```python
from build123d import *

# Parameters (mm, degrees)
SKETCH_W      = 300
SKETCH_H      = 300
PAD_DEPTH     = 30
SKETCH001_W   = 300
SKETCH001_H   = 300
SKETCH001_W_2 = 240
SKETCH001_H_2 = 240
PAD001_DEPTH  = 100


with BuildPart() as body:
    # Sketch → Pad (new body)
    with BuildSketch(Plane.XY):
        with Locations((150, 150)):
            Rectangle(SKETCH_W, SKETCH_H)
    extrude(amount=PAD_DEPTH)


with BuildPart() as body001:
    # Sketch001 (on Face6 of Pad) → Pad001 (new body)
    with BuildSketch(Plane.XY.offset(30)):
        with Locations((150, 150)):
            Rectangle(SKETCH001_W, SKETCH001_H)
        with Locations((150, 150)):
            Rectangle(SKETCH001_W_2, SKETCH001_H_2, mode=Mode.SUBTRACT)
    extrude(amount=PAD001_DEPTH)

    # Boolean: union Body
    add(body.part)


solid = body001.part
```
Input: part model. Units: mm. Frame: model coordinates. A direction names the side the tool comes from. Round coordinates to 2 decimals unless told otherwise and drop trailing zeros. Loops run counter-clockwise (first coordinate to the right, second up) from the corner with the lowest first, then second, coordinate; pieces in that order, holes last. Notation, with made-up numbers: (24, 86.25) -> (70, 86.25) arc R18 cw to (70, 118.25) -> close; hole circle Ø2 at (-7.75, 21.25). An arc over 180 degrees is marked (long way). One line per item, written item: value.
(1) Set-up query: faces 5 (the face through (30, 148, 79)), 6 (the face through (148, 0, 64)). Return all of +Z, -Z, +X, -X, +Y, -Y with unobstructed straight access to the full face (end or side cutting, diameter ignored); none if empty.
Geometry check:
face 5: +Z
face 6: +Z, -Z, +X, -X, -Y
(2) Pin query (flat end, axial travel): pin 1 (4 mm diameter, centred on x = 182, y = 217, fed in from +Z). Return the tip coordinate at first contact, or that it passes through.
Geometry check:
pin 1: z = 30
(3) Material intervals for line 1 (Y direction, x = 179, z = 89.5); line 2 (Z direction, x = 143.5, y = 48), sorted ascending. Write a range as [from, to].
Geometry check:
line 1: [0, 30], [270, 300]
line 2: [0, 30]
(4) Section B-B (x = 186). Return the cut outline in (y, z), plus the area to 3 significant figures.
Geometry check:
outline: (0, 0) -> (300, 0) -> (300, 130) -> (270, 130) -> (270, 30) -> (30, 30) -> (30, 130) -> (0, 130) -> close
area: 15,000 mm2
(5) Mould query, pull axis X, two halves, no side actions, for faces 1 (the face through (148, 152, 30)), 2 (the face through (270, 148, 79)), 3 (the face through (300, 148, 64)), 4 (the face through (0, 148, 64)). Classes: pulls with the +X half, pulls with the -X half, needs draft (parallel to the pull), parting line crosses it, or undercut.
Geometry check:
face 1: undercut
face 2: undercut
face 3: pulls with the +X half
face 4: pulls with the -X half
(6) Section A-A (z = 67). Return the cut outline in (x, y), plus the area to 3 significant figures.
Geometry check:
outline: (0, 0) -> (300, 0) -> (300, 300) -> (0, 300) -> close; hole (30, 30) -> (270, 30) -> (270, 270) -> (30, 270) -> close
area: 32,400 mm2
